Can you work these out from the model? Positions are in its coordinate system, mm. A direction names the side the tool comes from. Give positions to 0.01 mm unless a question says otherwise; leave off trailing zeros. Loops run counter-clockwise (first coordinate to the right, second up) from the corner with the lowest first, then second, coordinate; pieces in that order, holes last. Notation, with made-up numbers: (-20, -9.5) - (29, -9.5) arc R20 ccw to (29, 2.5) - close; hole circle Ø9 at (85.5, 26.25). An arc over 180 degrees is marked (long way). Write item = value, one per line.
from build123d import *

# Parameters (mm, degrees)
BOSS_EXTRUDE1_DEPTH = 30
SKETCH2_R           = 2
CUT_EXTRUDE1_DEPTH  = 2
SKETCH3_W           = 20
SKETCH3_H           = 53
CUT_EXTRUDE2_DEPTH  = 5


with BuildPart() as part:
    # Sketch1 → Boss-Extrude1 (new body)
    with BuildSketch(Plane.XY):
        with BuildLine():
            Line((-42, 31.5), (42, 31.5))
            ThreePointArc((42, 31.5), (45.535533906, 30.035533906), (47, 26.5))
            Line((47, 26.5), (47, -26.5))
            ThreePointArc((47, -26.5), (45.535533906, -30.035533906), (42, -31.5))
            Line((42, -31.5), (-42, -31.5))
            ThreePointArc((-42, -31.5), (-45.535533906, -30.035533906), (-47, -26.5))
            Line((-47, -26.5), (-47, 26.5))
            ThreePointArc((-47, 26.5), (-45.535533906, 30.035533906), (-42, 31.5))
        make_face()
    extrude(amount=BOSS_EXTRUDE1_DEPTH)

    # Sketch2 → Cut-Extrude1 (cut)
    with BuildSketch(Plane.XZ.offset(31.5)):
        with Locations((15, 10)):
            Circle(SKETCH2_R)
        with BuildLine():
            Line((-35, 12), (-27, 12))
            ThreePointArc((-27, 12), (-25, 10), (-27, 8))
            Line((-27, 8), (-35, 8))
            ThreePointArc((-35, 8), (-37, 10), (-35, 12))
        make_face()
        with BuildLine():
            Line((-19, 12), (-11, 12))
            ThreePointArc((-11, 12), (-9, 10), (-11, 8))
            Line((-11, 8), (-19, 8))
            ThreePointArc((-19, 8), (-21, 10), (-19, 12))
        make_face()
        with BuildLine():
            Line((-3, 12), (5, 12))
            ThreePointArc((5, 12), (7, 10), (5, 8))
            Line((5, 8), (-3, 8))
            ThreePointArc((-3, 8), (-5, 10), (-3, 12))
        make_face()
    extrude(amount=-CUT_EXTRUDE1_DEPTH, mode=Mode.SUBTRACT)

    # Sketch3 → Cut-Extrude2 (cut)
    with BuildSketch(Plane.ZY.offset(47)):
        with Locations((15, 0)):
            Rectangle(SKETCH3_W, SKETCH3_H)
    extrude(amount=-CUT_EXTRUDE2_DEPTH, mode=Mode.SUBTRACT)


solid = part.part
Q1. We'd pull the mould along Y, two halves only. Please class faces 1 (the flat face through (-45, 0, 25)), 2 (the cylindrical face through (13.526, -30.514, 11.352)), 3 (the flat face through (-45, 0, 5)), 4 (the flat face through (-31, -29.5, 10)): released by +Y, released by -Y, zero draft, split by the parting line, or undercut.
Output:
face_1 = undercut
face_2 = zero draft
face_3 = undercut
face_4 = released by -Y
Q2. I need wall thicknesses on L1, parallel to Z at x = 15, y = -30.9; L2, parallel to X at y = 16, z = 13.75; L3, parallel to X at y = 28, z = 15.25. Which ranges of each line are inside material? Lowest first, please.
Output:
L1 = 0 to 8, 12 to 30
L2 = -42 to 47
L3 = -46.77 to 46.77
Q3. Imagine slicing it at A-A, the plane y = -10. Write out the boundary of the cut face in (x, z).
Output:
outline = (-47, 0) - (47, 0) - (47, 30) - (-47, 30) - (-47, 25) - (-42, 25) - (-42, 5) - (-47, 5) - close
Q4. Imagine slicing it at C-C, the plane z = 10. Write out the boundary of the cut face in (x, y), then the cut area to 3 significant figures.
Output:
outline = (-47, -26.5) arc R5 ccw to (-42, -31.5) - (-37, -31.5) - (-37, -29.5) - (-25, -29.5) - (-25, -31.5) - (-21, -31.5) - (-21, -29.5) - (-9, -29.5) - (-9, -31.5) - (-5, -31.5) - (-5, -29.5) - (7, -29.5) - (7, -31.5) - (13, -31.5) - (13, -29.5) - (17, -29.5) - (17, -31.5) - (42, -31.5) arc R5 ccw to (47, -26.5) - (47, 26.5) arc R5 ccw to (42, 31.5) - (-42, 31.5) arc R5 ccw to (-47, 26.5) - (-42, 26.5) - (-42, -26.5) - close
area = 5,560 mm2
Q5. Which directions (+Z, -Z, +X, -X, +Y, -Y) give clear straight access to the entire face, cutting with the end or side of a thin tool? Please do faces 5 (the flat face through (47, 0, 15)), 6 (the flat face through (1, -29.5, 10)), 7 (the flat face through (-45, -26.5, 15)).
Output:
face_5 = +Z, -Z, +X, +Y, -Y
face_6 = -Y
face_7 = -X
Q6. For pin 1 (1.5 mm diameter, centred on x = -45, z = 19, fed in from +Y); pin 2 (1.2 mm diameter, centred on x = 16, z = 9.5, fed in from -Y); pin 3 (16 mm diameter, centred on y = -6.5, z = 16, fed in from -X), each with a flat end and sliding along its axis, tell me the tip position at first contact or that it passes through.
Output:
pin_1 = 30.97
pin_2 = -29.5
pin_3 = -42
Q7. Imagine slicing it at B-B, the plane z = 19. Write out the boundary of the cut face in (x, y), then the cut area to 3 significant figures.
Output:
outline = (-47, -26.5) arc R5 ccw to (-42, -31.5) - (42, -31.5) arc R5 ccw to (47, -26.5) - (47, 26.5) arc R5 ccw to (42, 31.5) - (-42, 31.5) arc R5 ccw to (-47, 26.5) - (-42, 26.5) - (-42, -26.5) - close
area = 5,640 mm2
